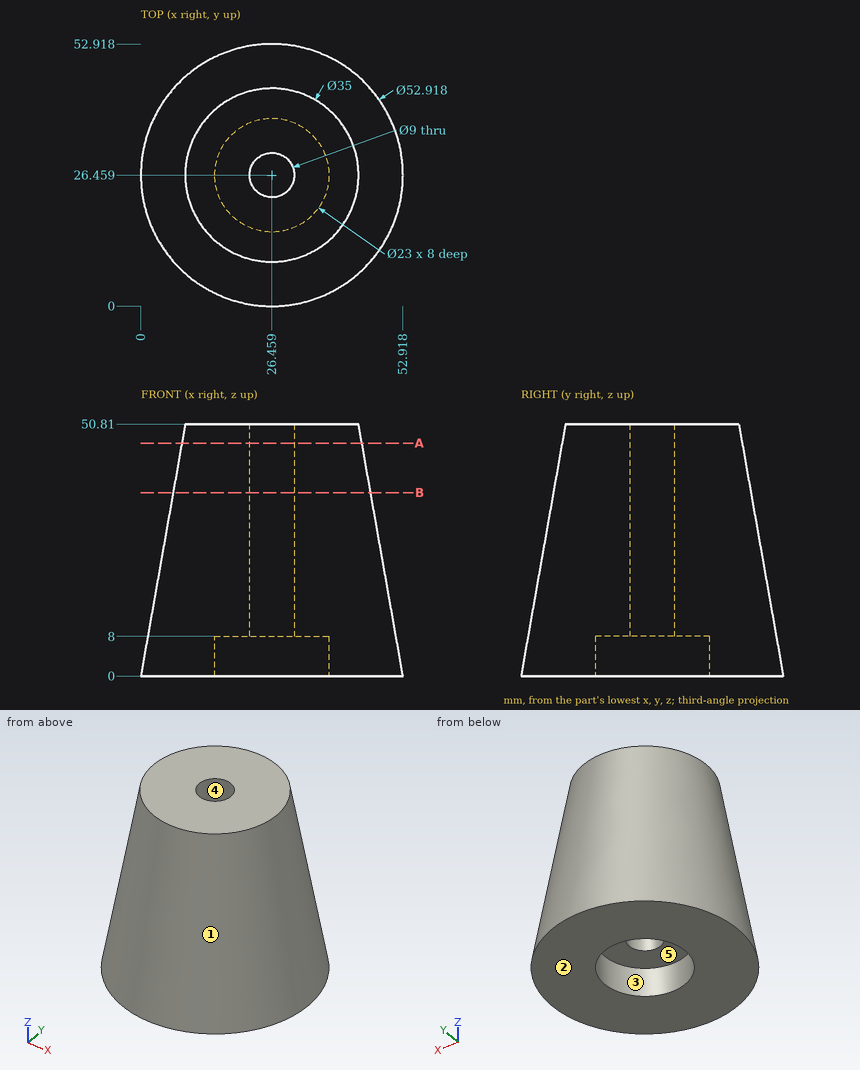
Geometry: see drawing. Coordinates: mm, zero at the bounding-box minimum. A direction names the side the tool comes from. Give positions to 0.01 mm unless a question says otherwise; leave off trailing zeros. Order: outer loops, then holes, each group sorted by start corner. A loop starts at its lowest first (then second) coordinate and runs counter-clockwise, first axis right, second up. Notation, with made-up numbers: (66.5, 14) - (114.5, 14) arc R34 cw to (114.5, 52) - close; hole circle Ø7 at (-33.75, 3). An arc over 180 degrees is marked (long way). One line per item, written item: value.
1. Pin query (flat end, axial travel): pin 1 Ø12 at (x, z) = (13, 28) entering from -Y; pin 2 Ø10 at (x, z) = (33.5, 34) entering from -Y (1 decimal); pin 3 Ø3 at (x, z) = (36.5, 35) entering from -Y. Return the tip coordinate at first contact, or that it passes through.
Determined:
pin 1: y = 6.01
pin 2: y = 5.7
pin 3: y = 8
2. Cut plane A-A, the plane z = 47. Output: boundary loops of the cut face in (x, y), and give its area (3 significant figures).
Determined:
outline: circle Ø36.34 at (26.46, 26.46); hole circle Ø9 at (26.46, 26.46)
area: 974 mm2
3. Line query: probe 1 along Z at (x, y) = (27, 20); probe 2 along X at (y, z) = (30, 42) (1 decimal); probe 3 along Y at (x, z) = (46.5, 16.5) (1 decimal). Output: solid intervals per line, ascending.
Determined:
probe 1: 8 to 50.81
probe 2: 7.7 to 23.7, 29.2 to 45.2
probe 3: 14.1 to 38.8
4. Draft query along X for the marked faces 1, 2 and 3. Return one class per face: released by +X, released by -X, zero draft, split by the parting line, or undercut.
Determined:
face 1: split by the parting line
face 2: zero draft
face 3: undercut
5. Cut plane B-B, the plane z = 37. Output: boundary loops of the cut face in (x, y) (1 decimal).
Determined:
outline: circle Ø39.9 at (26.5, 26.5); hole circle Ø9 at (26.5, 26.5)
6. Reachability of the marked faces 4 and 5 from +Z, -Z, +X, -X, +Y, -Y: full face, straight path, thin tool, end or side. Return the list, or none.
Determined:
face 4: +Z, -Z
face 5: -Z
